The drawing under review shows one solid part. Ordinate dimensions are in mm from its lowest x, y, z. Coordinates: 2 decimals unless noted, no trailing zeros. Loops run counter-clockwise (first coordinate to the right, second up) from the corner with the lowest first, then second, coordinate; pieces in that order, holes last. Notation, with made-up numbers: (-8.5, 88) - (20.5, 88) arc R21 ccw to (20.5, 110) - close; hole circle Ø1 at (76.5, -27). An arc over 180 degrees is marked (long way). Answer as a JSON object with one key per item and string values. Group by question number.
Item 1: We need section B-B (y = 6). Give the boundary of the cut face in (x, z) (3 decimals), then the cut area to 3 significant figures.
Item 2: We need section C-C (x = 16). Give the boundary of the cut face in (y, z).
Item 3: To check wall thickness, follow line 1 (X direction, y = 30, z = 12.5); line 2 (X direction, y = 2.5, z = 7.5) (3 decimals); line 3 (Z direction, x = 16.5, y = 18.5). State the ranges of each line that lie inside material, in increasing order.
Item 4: We need section D-D (z = 16.5). Give the boundary of the cut face in (x, y), then the cut area to 3 significant figures.
Item 5: Clearance check with flat-ended pins moving along their axes: pin 1 (10 mm diameter, centred on x = 28, y = 19, fed in from +Z); pin 2 (2.5 mm diameter, centred on x = 33.6, y = 8.44, fed in from +Z). State where each tip first meets the part, or that it passes through.
Item 6: Mouldability with a two-part tool opening along X and no side actions: class the marked faces 1, 2 and 3 as released by +X, released by -X, zero draft, split by the parting line, or undercut.
Item 7: We need section A-A (z = 7.62). Give the boundary of the cut face in (x, y), then the cut area to 3 significant figures.
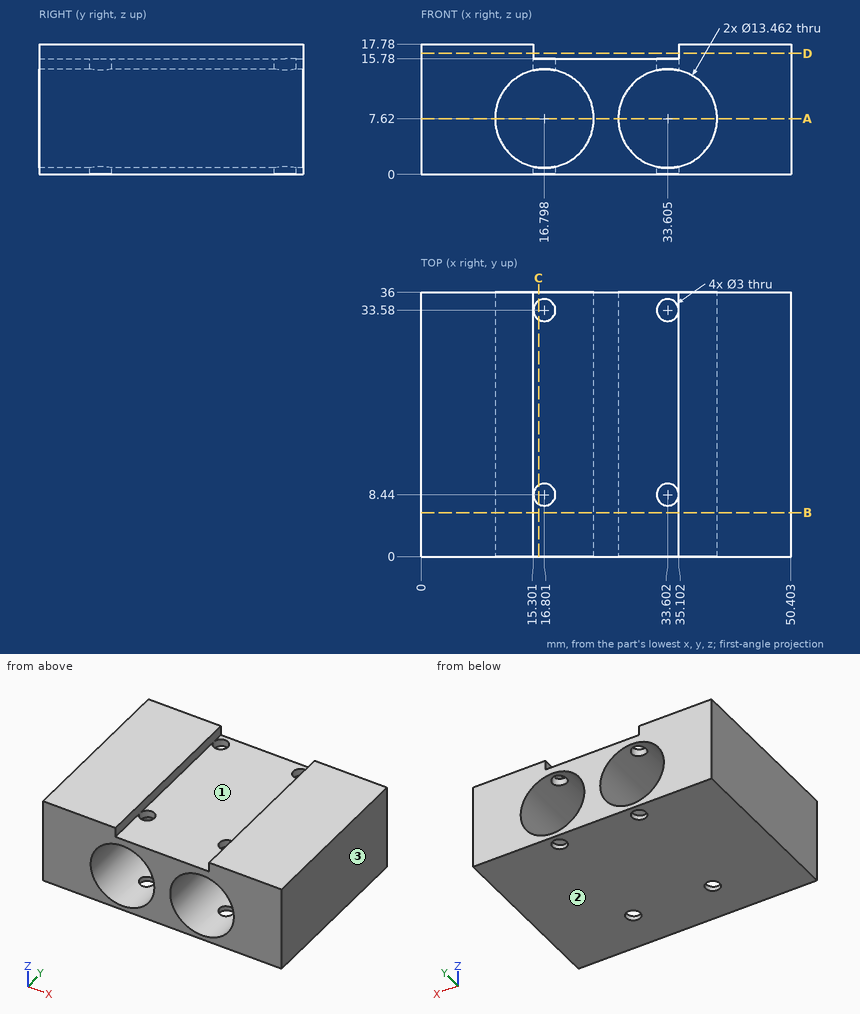
Check sheet entries:
{
 "1": {"outline": "(0, 0) - (50.403, 0) - (50.403, 17.78) - (35.102, 17.78) - (35.102, 15.78) - (15.301, 15.78) - (15.301, 17.78) - (0, 17.78) - close; hole circle Ø13.462 at (16.798, 7.62); hole circle Ø13.462 at (33.605, 7.62)", "area": "572 mm2"},
 "2": {"outline": "(0, 0) - (7.17, 0) - (7.17, 0.94) - (0, 0.94) - close; (0, 14.3) - (7.17, 14.3) - (7.17, 15.78) - (0, 15.78) - close; (9.71, 0) - (32.31, 0) - (32.31, 0.94) - (9.71, 0.94) - close; (9.71, 14.3) - (32.31, 14.3) - (32.31, 15.78) - (9.71, 15.78) - close; (34.85, 0) - (36, 0) - (36, 0.94) - (34.85, 0.94) - close; (34.85, 14.3) - (36, 14.3) - (36, 15.78) - (34.85, 15.78) - close"},
 "3": {"line 1": "x = 0 to 12.16, 21.43 to 28.97, 38.24 to 50.4", "line 2": "x = 0 to 10.068, 23.528 to 26.875, 40.335 to 50.403", "line 3": "z = 0 to 0.9, 14.34 to 15.78"},
 "4": {"outline": "(0, 0) - (15.3, 0) - (15.3, 36) - (0, 36) - close; (35.1, 0) - (50.4, 0) - (50.4, 36) - (35.1, 36) - close", "area": "1,100 mm2"},
 "5": {"pin 1": "stops at z = 15.78", "pin 2": "passes through"},
 "6": {"face 1": "undercut", "face 2": "zero draft", "face 3": "released by +X"},
 "7": {"outline": "(0, 0) - (10.07, 0) - (10.07, 36) - (0, 36) - close; (23.53, 0) - (26.87, 0) - (26.87, 36) - (23.53, 36) - close; (40.34, 0) - (50.4, 0) - (50.4, 36) - (40.34, 36) - close", "area": "845 mm2"}
}
